Source: CAD feature listing. Evaluate the final solid. Frame: model axes, mm. Face numbers are marked on the shaded views. A direction names the side the tool comes from. Round coordinates to 2 decimals unless told otherwise and drop trailing zeros. Order: outer loops, then holes, each group sorted by start corner. A loop starts at its lowest first (then second) coordinate and runs counter-clockwise, first axis right, second up. Notation, with made-up numbers: (47, 44.25) -> (73, 44.25) arc R12 ccw to (73, 55.25) -> close; hole circle Ø8 at (10.25, 57.5). An arc over 180 degrees is marked (long way). Answer as CSV lines item,"result".
Autodesk Inventor part; units mm, degrees
ref_plane "YZ Plane" through (0, 0, 0) normal (1, 0, 0) x (0, 1, 0)
ref_plane "XZ Plane" through (0, 0, 0) normal (0, 1, 0) x (-1, 0, 0)
ref_plane "XY Plane" through (0, 0, 0) normal (0, 0, 1) x (1, 0, 0)
sketch "Sketch1" plane through (0, 0, 0) normal (0, 1, 0) x (-1, 0, 0)
  circle A0 centre (0, 0) radius 4.5
  circle A1 centre (0, 0) radius 25
  circle A2 centre (0, 0) radius 7.5
  circle A3 centre (0, 0) radius 21
  line L0 (0, 0) -> (25, 0)
  line L1 (22.5, 2) -> (22.5, -2)
  line L2 (22.5, -2) -> (2.5, -2)
  line L3 (2.5, -2) -> (2.5, 2)
  line L4 (2.5, 2) -> (22.5, 2)
  line L5 (22.5, 2) -> (2.5, -2) construction
  line L6 (22.5, -2) -> (2.5, 2) construction
  line L7 (5.0508, 22.0168) -> (8.855, 20.7807)
  line L8 (-1.1296, 2.9957) -> (5.0508, 22.0168)
  line L9 (8.855, 20.7807) -> (2.6747, 1.7596)
  line L10 (2.6747, 1.7596) -> (-1.1296, 2.9957)
  line L11 (-19.3785, 11.6071) -> (-17.0273, 14.8432)
  line L12 (-3.1981, -0.1486) -> (-19.3785, 11.6071)
  line L13 (-17.0273, 14.8432) -> (-0.847, 3.0875)
  line L14 (-0.847, 3.0875) -> (-3.1981, -0.1486)
  line L15 (-17.0273, -14.8432) -> (-19.3785, -11.6071)
  line L16 (-0.847, -3.0875) -> (-17.0273, -14.8432)
  line L17 (-19.3785, -11.6071) -> (-3.1981, 0.1486)
  line L18 (-3.1981, 0.1486) -> (-0.847, -3.0875)
  line L19 (8.855, -20.7807) -> (5.0508, -22.0168)
  line L20 (2.6747, -1.7596) -> (8.855, -20.7807)
  line L21 (5.0508, -22.0168) -> (-1.1296, -2.9957)
  line L22 (-1.1296, -2.9957) -> (2.6747, -1.7596)
  point P0 (12.5, 0)
  point P1 (7.2284, -2)
  point P2 (20.9045, -2)
  point P3 (8.362, -19.2634)
  point P4 (4.1358, -6.2566)
  point P5 (7.2284, 2)
  point P6 (4.1358, 6.2566)
  point P7 (8.362, 19.2634)
  point P8 (20.9045, 2)
  point P9 (0.3316, 7.4927)
  point P10 (-4.6723, 5.8668)
  point P11 (-15.7366, 13.9054)
  point P12 (4.5577, 20.4994)
  point P13 (-4.6723, -5.8668)
  point P14 (0.3316, -7.4927)
  point P15 (4.5577, -20.4994)
  point P16 (-15.7366, -13.9054)
  point P17 (-7.0235, 2.6307)
  point P18 (-7.0235, -2.6307)
  point P19 (-18.0877, -10.6693)
  point P20 (-18.0877, 10.6693)
  dimension "d1" = 50
  dimension "d0" = 9
  dimension "d2" = 3
  dimension "d3" = 4
  dimension "d4" = 4
  dimension "d5" = 20
  dimension "d8" = 360
extrude "Extrusion1" add sketch "Sketch1" along normal blind 6 contours L0 A2 L2 A0 | A0 L4 A2 L0 | A0 L9 A2 L4 | L2 A2 L20 A0 | L0 A3 L2 A2 | A2 L4 A3 L0 | A0 L8 A2 L9 | L20 A2 L21 A0 | L0 L1 L2 A3 | A3 L4 L1 L0 | A0 L13 A2 L8 | A2 L8 A3 L9 | A1 | L21 A2 L16 A0 | L20 A3 L21 A2 | A0 L12 A2 L13 | A3 L8 L7 L9 | L16 A2 L17 A0 | L20 L19 L21 A3 | A0 L17 A2 L12 | A2 L12 A3 L13 | L16 A3 L17 A2 | A3 L12 L11 L13 | L16 L15 L17 A3
fillet "Fillet1" radius 2 4 edges at (-8.362, 3, 19.2634) (-20.9045, 3, 2) (-7.2284, 3, 2) (-4.1358, 3, 6.2566)
pattern_circular "Circular Pattern1" count 5 over 360 about axis through (0, 0, 0) along (0, 1, 0) of "Fillet1"
properties part number "8_6mm"
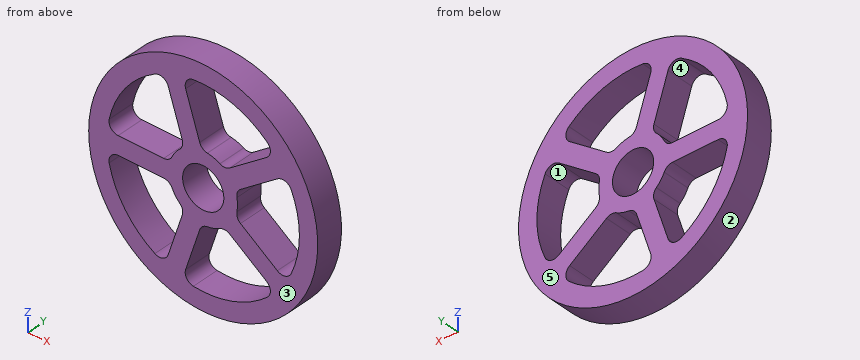
1. Section query A-A on z = 0. Return loops of the section in (x, y).
Results below:
outline,"(-25, 0) -> (-4.5, 0) -> (-4.5, 6) -> (-25, 6) -> close; (4.5, 0) -> (7.5, 0) -> (7.5, 6) -> (4.5, 6) -> close; (21, 0) -> (25, 0) -> (25, 6) -> (21, 6) -> close"
2. Section query C-C on x = -14. Return loops of the section in (y, z).
Results below:
outline,"(0, -20.71) -> (6, -20.71) -> (6, -15.65) -> (0, -15.65) -> close; (0, -2) -> (6, -2) -> (6, 2) -> (0, 2) -> close; (0, 15.65) -> (6, 15.65) -> (6, 20.71) -> (0, 20.71) -> close"
3. Mould query, pull axis X, two halves, no side actions, for the marked faces 1, 2 and 3. Classes: released by +X, released by -X, zero draft, split by the parting line, or undercut.
Results below:
face 1,"undercut"
face 2,"split by the parting line"
face 3,"zero draft"
4. Section query B-B on x = 0. Return loops of the section in (y, z).
Results below:
outline,"(0, -25) -> (6, -25) -> (6, -21) -> (0, -21) -> close; (0, -7.79) -> (6, -7.79) -> (6, -4.5) -> (0, -4.5) -> close; (0, 4.5) -> (6, 4.5) -> (6, 7.79) -> (0, 7.79) -> close; (0, 21) -> (6, 21) -> (6, 25) -> (0, 25) -> close"
5. Line query: L1, parallel to Z at x = -12.5, y = 1.2; L2, parallel to X at y = 1.3, z = 4; L3, parallel to Z at x = 10.5, y = 2.6. Output: solid intervals per line, ascending. Write a range as [from, to].
Results below:
L1,"[-21.65, -16.87], [-2, 2], [16.87, 21.65]"
L2,"[-24.68, -20.57], [-6.34, -2.06], [2.06, 8.91], [20.62, 24.68]"
L3,"[-22.69, -18.19], [-10.1, -5.16], [5.16, 10.1], [18.19, 22.69]"
6. Pin query (flat end, axial travel): pin 1 (1.5 mm diameter, centred on y = 1.5, z = 7, fed in from +X); pin 2 (10 mm diameter, centred on x = -2.5, z = 19, fed in from +Y); pin 3 (3 mm diameter, centred on y = 1.5, z = -6.5, fed in from -X). Return the tip coordinate at first contact, or that it passes through.
Results below:
pin 1,"x = 24.21"
pin 2,"y = 6"
pin 3,"x = -24.49"
7. Reachability of the marked faces 4 and 5 from +Z, -Z, +X, -X, +Y, -Y: full face, straight path, thin tool, end or side. Return the list, or none.
Results below:
face 4,"+Y, -Y"
face 5,"+Z, -Z, +X, -X, +Y"
8. Section query D-D on y = 1.3. Give the number of separate pieces and of enclosed holes in the cut face, and give its area (3 significant figures).
Results below:
separate pieces,"1"
enclosed holes,"6"
area,"978 mm2"
